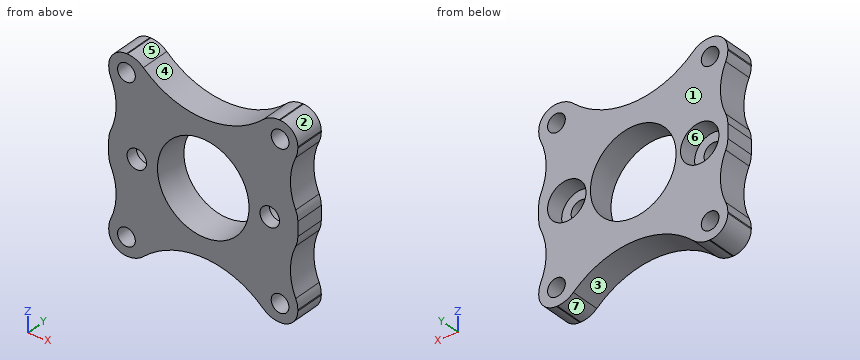
```python
from build123d import *

# Parameters (mm, degrees)
F0_R           = 1.5
F0_R_2         = 7.25
F1_DEPTH       = 5
F2_R           = 3
F3_SIZE2       = 4.99999
F3_SIZE        = 0.49999
F4_D           = 3.3
F4_CBORE_D     = 6.5
F4_CBORE_DEPTH = 3
F5_R           = 4


# Not quite as in the source:
# - a fillet or chamfer is up to 0.001 mm smaller than in the source, because OpenCascade refuses the exact size


with BuildPart() as f1:
    # F0 (on Front) → F1 (new body)
    with BuildSketch(Plane.XZ):
        with BuildLine():
            Line((11.1803398875, -16), (16, -16))
            Line((16, -16), (16, -11.8509778157))
            ThreePointArc((16, -11.8509778157), (14.7445991464, -7), (16, -2.1490221843))
            Line((16, -2.1490221843), (16, 2.1490221843))
            ThreePointArc((16, 2.1490221843), (14.7445991464, 7), (16, 11.8509778157))
            Line((16, 11.8509778157), (16, 16))
            Line((16, 16), (11.1803398875, 16))
            ThreePointArc((11.1803398875, 16), (0, 11), (-11.1803398875, 16))
            Line((-11.1803398875, 16), (-16, 16))
            Line((-16, 16), (-16, 11.8509778157))
            ThreePointArc((-16, 11.8509778157), (-14.7445991464, 7), (-16, 2.1490221843))
            Line((-16, 2.1490221843), (-16, -2.1490221843))
            ThreePointArc((-16, -2.1490221843), (-14.7445991464, -7), (-16, -11.8509778157))
            Line((-16, -11.8509778157), (-16, -16))
            Line((-16, -16), (-11.1803398875, -16))
            ThreePointArc((-11.1803398875, -16), (0, -11), (11.1803398875, -16))
        make_face()
        with Locations((-13, -13)):
            Circle(F0_R, mode=Mode.SUBTRACT)
        with Locations((13, -13)):
            Circle(F0_R, mode=Mode.SUBTRACT)
        with Locations((-13, 13)):
            Circle(F0_R, mode=Mode.SUBTRACT)
        Circle(F0_R_2, mode=Mode.SUBTRACT)
        with Locations((13, 13)):
            Circle(F0_R, mode=Mode.SUBTRACT)
    extrude(amount=F1_DEPTH)

    # F2
    f2_edges = [f1.edges().sort_by_distance(p)[0] for p in [
        (-16, -2.5, 16),
        (16, -2.5, 16),
        (16, -2.5, -16),
        (-16, -2.5, -16),
    ]]
    fillet(f2_edges, radius=F2_R)

    # F3 (size 0.5 and 5 in the source; OpenCascade refuses exactly that, so slightly less here)
    f3_edges = [f1.edges().sort_by_distance(p)[0] for p in [
        (-7.25, -5, 0),
    ]]
    f3_side = f1.faces().sort_by_distance((-15.547452, -5, -12.425489))[0]
    chamfer(f3_edges, length=F3_SIZE, length2=F3_SIZE2, reference=f3_side)

    # F4 (through all)
    with Locations(Plane(origin=(0, 0, 0), x_dir=(1, 0, 0), z_dir=(0, 1, 0))):
        with Locations((11.25, 0), (-11.25, 0)):
            CounterBoreHole(F4_D / 2, F4_CBORE_D / 2, F4_CBORE_DEPTH)

    # F5
    f5_edges = [f1.edges().sort_by_distance(p)[0] for p in [
        (-16, -2.5, -2.149022),
        (-16, -2.5, 2.149022),
        (-16, -2.5, 13),
        (11.18034, -2.5, 16),
        (16, -2.5, 2.149022),
        (16, -2.5, -2.149022),
        (11.18034, -2.5, -16),
        (-16, -2.5, -11.850978),
        (-11.18034, -2.5, -16),
        (-16, -2.5, 11.850978),
        (16, -2.5, -11.850978),
        (-11.18034, -2.5, 16),
        (16, -2.5, 11.850978),
    ]]
    fillet(f5_edges, radius=F5_R)


solid = f1.part
```
The listing builds one solid part. Answer for the finished solid, in the listing's coordinates (mm). Face numbers are marked on the shaded views. A direction names the side the tool comes from. Give positions to 0.01 mm unless a question says otherwise; leave off trailing zeros. Order: outer loops, then holes, each group sorted by start corner. A loop starts at its lowest first (then second) coordinate and runs counter-clockwise, first axis right, second up. Notation, with made-up numbers: (52.5, 77) - (95.5, 77) arc R20 cw to (95.5, 102) - close; hole circle Ø2 at (21.25, -24.5). An arc over 180 degrees is marked (long way). Use one line per item in the form item = value. Start each with the question number.
(1) Consider line 1 (X direction, y = -4.5, z = 1); line 2 (X direction, y = -0.9, z = 1.5); line 3 (Z direction, x = 12, y = -2.15). Determine where each line is inside the solid, lowest interval first. Write a range as from..to.
(2) A cutting plane is placed at C-C, the plane y = -1.75. State how many separate pieces and enclosed holes the cut face has, then the cut area to 3 significant figures.
(3) Flat-ended cylindrical pins translate along their axes: pin 1 Ø12 at (x, z) = (5.5, 10) entering from +Y; pin 2 Ø1 at (x, y) = (10.5, -3.5) entering from -Z; pin 3 Ø8.5 at (x, z) = (0, 0) entering from +Y; pin 4 Ø6 at (x, z) = (-11.25, 0) entering from +Y. Find the tip coordinate at first contact, or state that the pin passes through.
(4) The mould has two halves that part along X. Classify the marked faces 1, 2, 3 and 4: released by +X, released by -X, zero draft, split by the parting line, or undercut.
(5) For the marked faces 5, 6 and 7, determine the directions among +Z, -Z, +X, -X, +Y, -Y from which every point of the face is accessible in a straight line to the end or side of a thin tool.
(6) A cutting plane is placed at B-B, the plane x = 14. Write down the section's boundary in (y, z), then the cut area to 3 significant figures.
(7) A cutting plane is placed at D-D, the plane x = -8.5. Write down the section's boundary in (y, z).
Ans:
q1.line_1 = -16..-12.56, -9.94..-7.63, 7.63..9.94, 12.56..16
q1.line_2 = -15.99..-14.13, -8.37..-7.19, 7.19..8.37, 14.13..15.99
q1.line_3 = -15.91..-14.12, -11.88..-3.16, 3.16..11.88, 14.12..15.91
q2.separate_pieces = 1
q2.enclosed_holes = 7
q2.area = 559 mm^2
q3.pin_1 = 0
q3.pin_2 = -15.55
q3.pin_3 = through
q3.pin_4 = -3
q4.face_1 = zero draft
q4.face_2 = released by +X
q4.face_3 = undercut
q4.face_4 = undercut
q5.face_5 = +Z, +Y, -Y
q5.face_6 = +Y
q5.face_7 = -Z, +Y, -Y
q6.outline = (-5, -15.83) - (0, -15.83) - (0, -14.12) - (-5, -14.12) - close; (-5, -11.88) - (0, -11.88) - (0, -1.73) - (-3, -1.73) - (-3, 1.73) - (0, 1.73) - (0, 11.88) - (-5, 11.88) - close; (-5, 14.12) - (0, 14.12) - (0, 15.83) - (-5, 15.83) - close
q6.area = 126 mm^2
q7.outline = (-5, -13.64) - (0, -13.64) - (0, -1.73) - (-3, -1.73) - (-3, 1.73) - (0, 1.73) - (0, 13.64) - (-5, 13.64) - close
